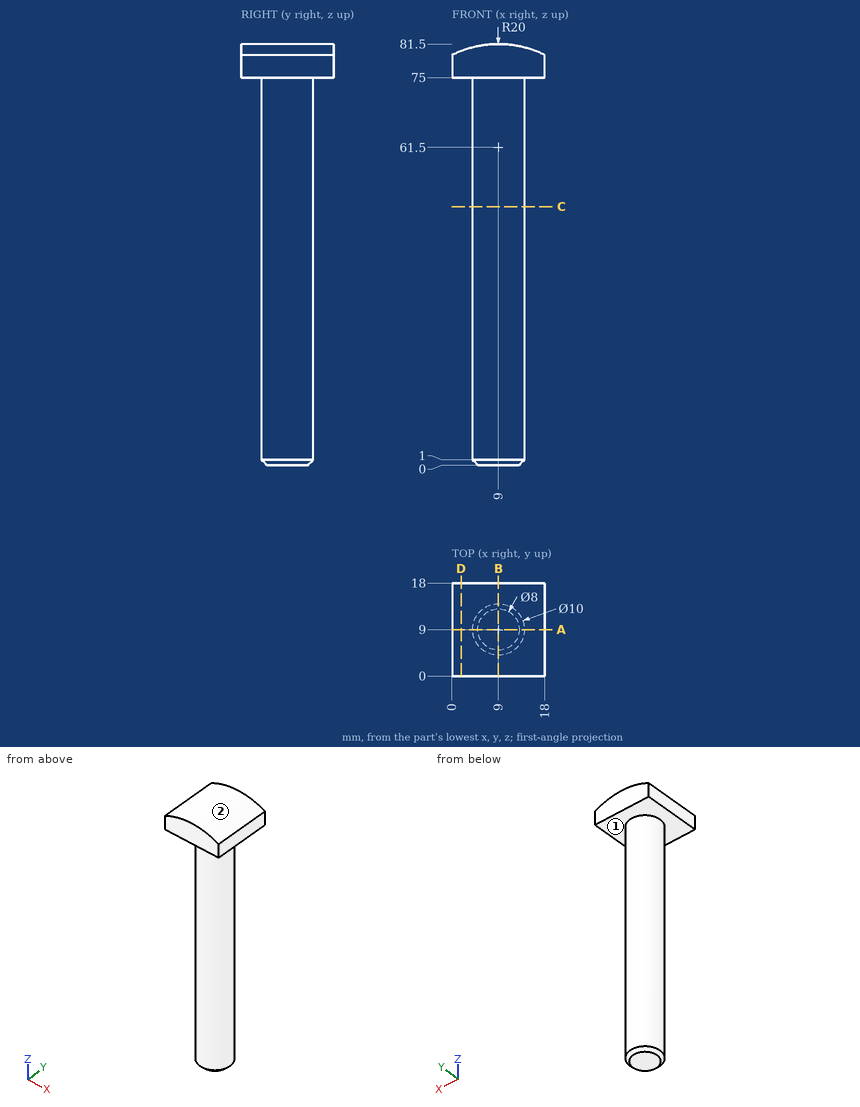
Can you work these out from the drawing? Everything is in mm from the part's minimum corner. A direction names the side the tool comes from. Give positions to 0.01 mm unless a question says otherwise; leave off trailing zeros. Order: outer loops, then holes, each group sorted by start corner. A loop starts at its lowest first (then second) coordinate and runs counter-clockwise, first axis right, second up.
1. Suppose I cut it at B-B (x = 9). List the corners of the cut face in (y, z) for me, plus the area to 3 significant figures.
2. For the marked faces 1 and 2, which set-ups out of +Z, -Z, +X, -X, +Y, -Y let a thin tool reach every point of the face, with its end or its side?
3. Suppose I cut it at C-C (z = 50). List the corners of the cut face in (x, y) for me.
4. Suppose I cut it at D-D (x = 1.75). List the corners of the cut face in (y, z) for me.
5. I need wall thicknesses on L1, parallel to Y at x = 6, z = 48; L2, parallel to Z at x = 8.75, y = 10.5; L3, parallel to Z at x = 2.75, y = 10. Which ranges of each line are inside material? Lowest first, please.
6. Suppose I cut it at A-A (y = 9). List the corners of the cut face in (x, z) for me.
7. Will these pins go through, and if not, where does the flat tip stop? P1, Ø8, axis at x = 5, z = 19, coming from the -Y side; P2, Ø1.5, axis at x = 2, z = 29, coming from the +Y side; P3, Ø10, axis at y = 7.5, z = 25.5, coming from the +X side; P4, Ø8, axis at y = 8, z = 22, coming from the -X side.
Solved:
1. outline: (0, 75) - (4, 75) - (4, 1) - (5, 0) - (13, 0) - (14, 1) - (14, 75) - (18, 75) - (18, 81.5) - (0, 81.5) - close
1. area: 866 mm2
2. face 1: -Z
2. face 2: +Z, +Y, -Y
3. outline: circle Ø10 at (9, 9)
4. outline: (0, 75) - (18, 75) - (18, 80.14) - (0, 80.14) - close
5. L1: y = 5 to 13
5. L2: z = 0 to 81.5
5. L3: z = 75 to 80.5
6. outline: (0, 75) - (4, 75) - (4, 1) - (5, 0) - (13, 0) - (14, 1) - (14, 75) - (18, 75) - (18, 79.36) arc R20 ccw to (0, 79.36) - close
7. P1: stops at y = 4
7. P2: passes through
7. P3: stops at x = 14
7. P4: stops at x = 4
